from build123d import *

# Parameters (mm, degrees)
BOSS_EXTRUDE1_DEPTH     = 40
BOSS_EXTRUDE2_START     = 30
SKETCH2_R               = 1.25
BOSS_EXTRUDE2_DEPTH     = 10
CUT_EXTRUDE1_START      = -30
SKETCH3_W               = 5
SKETCH3_H               = 5
CUT_EXTRUDE1_DEPTH      = 10
CUT_EXTRUDE2_DEPTH      = 100.624294226
CUT_EXTRUDE2_DEPTH_BACK = 100.624294226
SKETCH4_R               = 1.25
FILLET1_R               = 2.5


with BuildPart() as part:
    # Sketch1 → Boss-Extrude1 (new, symmetric)
    with BuildSketch(Plane.XY):
        Polygon((0, 0), (90, 0), (90, 15), (85, 15), (85, 5), (0, 5), align=None)
    extrude(amount=BOSS_EXTRUDE1_DEPTH, both=True)

    # Sketch2 → Boss-Extrude2 (add)
    with BuildSketch(Plane.XY.offset(BOSS_EXTRUDE2_START)):
        with BuildLine():
            Line((0, 5), (-2.5, 5))
            ThreePointArc((-2.5, 5), (-5, 2.5), (-2.5, 0))
            Line((-2.5, 0), (0, 0))
            Line((0, 0), (0, 5))
        make_face()
        with Locations((-2.5, 2.5)):
            Circle(SKETCH2_R, mode=Mode.SUBTRACT)
    boss_extrude2 = extrude(amount=BOSS_EXTRUDE2_DEPTH)

    # Mirror2: Boss-Extrude2 across plane
    add(boss_extrude2.mirror(Plane.XY))

    # Sketch3 → Cut-Extrude1 (cut)
    with BuildSketch(Plane.XY.offset(CUT_EXTRUDE1_START)):
        with Locations((87.5, 12.5)):
            Rectangle(SKETCH3_W, SKETCH3_H)
    cut_extrude1 = extrude(amount=-CUT_EXTRUDE1_DEPTH, mode=Mode.SUBTRACT)

    # Mirror3: Cut-Extrude1 across plane
    add(cut_extrude1.mirror(Plane.XY), mode=Mode.SUBTRACT)

    # Sketch4 → Cut-Extrude2 (cut, two sides: drawn at the far end of the back side and taken through both)
    with BuildSketch(Plane.XY.offset(-CUT_EXTRUDE2_DEPTH_BACK)):
        with Locations((87.5, 12.5)):
            Circle(SKETCH4_R)
    extrude(amount=CUT_EXTRUDE2_DEPTH + CUT_EXTRUDE2_DEPTH_BACK, mode=Mode.SUBTRACT)

    # Fillet1
    fillet1_edges = [part.edges().sort_by_distance(p)[0] for p in [
        (85, 15, 0),
        (90, 15, 0),
    ]]
    fillet(fillet1_edges, radius=FILLET1_R - 0.0001)  # a hair under: the kernel refuses the full size


solid = part.part
The model under review builds one solid part; all positions refer to its coordinate system, in mm. A direction names the side the tool comes from. Round coordinates to 2 decimals unless told otherwise and drop trailing zeros. Write each loop counter-clockwise with the first axis right and the second up, starting at its lowest first coordinate (ties: lowest second). Pieces come first, ordered by that corner, then holes. Notation, with made-up numbers: M 67.25,54 L 74.25,54 A30 cw 74.25,78 Z; hole C 31.5,-1 d5. An arc over 180 degrees is marked long. Use a Markdown table: item, result. Add a question column.
Q1. The part is to be moulded in two halves that separate along Y. For faces 1 (the face through (42, 5, 1)), 2 (the face through (43, 0, 1)), 3 (the face through (86, 12, -30)), 4 (the face through (-1.31, 2.88, 34.93)), say which applies: pulls with the +Y half, pulls with the -Y half, needs draft (parallel to the pull), parting line crosses it, or undercut.
Q2. To check wall thickness, follow line 1 (X direction, y = 12.5, z = 15); line 2 (Y direction, x = 28, z = -25.5); line 3 (X direction, y = 6.75, z = -2.5). State the ranges of each line that lie inside material, in increasing order.
Q3. We need section C-C, the plane x = 46.5. State the section outline as (y, z) points, plus the area to 3 significant figures.
Q4. Insertion check: pin 1 (5.5 mm diameter, centred on x = 87, z = 35.5, fed in from +Y); pin 2 (6 mm diameter, centred on x = 22, z = 18.5, fed in from +Y); pin 3 (4 mm diameter, centred on x = -2.5, y = 3, fed in from -Z); pin 4 (4 mm diameter, centred on y = 1.5, z = -11, fed in from -X). Each pin has a flat end and moves straight along its axis. Give the tip position at first contact, or say it passes through.
Q5. Machinability: for faces 5 (the face through (86, 12, 30)), 6 (the face through (0, 3, 0)), 7 (the face through (85, 9, 1)), which of the approach directions +Z, -Z, +X, -X, +Y, -Y give a long, thin tool a straight path to every point of the face, cutting with its end or side? Answer none if there is none.
Q6. We need section A-A, the plane y = 2.5. State the section outline as (x, z) points, plus the area to 3 significant figures.
Findings below:
| question | item | result |
|---|---|---|
| 1 | face 1 | pulls with the +Y half |
| 1 | face 2 | pulls with the -Y half |
| 1 | face 3 | needs draft |
| 1 | face 4 | undercut |
| 2 | line 1 | x = 85 to 86.25, 88.75 to 90 |
| 2 | line 2 | y = 0 to 5 |
| 2 | line 3 | x = 85 to 90 |
| 3 | outline | M 0,-40 L 5,-40 L 5,40 L 0,40 Z |
| 3 | area | 400 mm² |
| 4 | pin 1 | stops at y = 10 |
| 4 | pin 2 | stops at y = 5 |
| 4 | pin 3 | stops at z = -40 |
| 4 | pin 4 | stops at x = 0 |
| 5 | face 5 | +Z, +X, -X, +Y |
| 5 | face 6 | -X, +Y, -Y |
| 5 | face 7 | +Z, -Z, -X, +Y |
| 6 | outline | M -5,-40 L -3.75,-40 L -3.75,-30 L -5,-30 Z; M -5,30 L -3.75,30 L -3.75,40 L -5,40 Z; M -1.25,-40 L 90,-40 L 90,40 L -1.25,40 L -1.25,30 L 0,30 L 0,-30 L -1.25,-30 Z |
| 6 | area | 7,250 mm² |
